```python
from build123d import *

# Parameters (mm, degrees)
SKETCH1_R           = 1.4
BOSS_EXTRUDE1_DEPTH = 0.8


with BuildPart() as part:
    # Sketch1 → Boss-Extrude1 (new, symmetric)
    with BuildSketch(Plane(origin=(0, 0, 0), x_dir=(0, 0, -1), z_dir=(1, 0, 0))):
        with BuildLine():
            Line((-35.297434934, -41.688153), (-20.809434934, -41.688153))
            Line((-20.809434934, -41.688153), (-20.809434934, -39.097053))
            Line((-20.809434934, -39.097053), (14.496565066, -39.097053))
            Line((14.496565066, -39.097053), (14.496565066, -41.688153))
            Line((14.496565066, -41.688153), (34.592039339, -41.688153))
            ThreePointArc((34.592039339, -41.688153), (38.127573245, -40.223686906), (39.592039339, -36.688153))
            Line((39.592039339, -36.688153), (39.592039339, 35.784769822))
            ThreePointArc((39.592039339, 35.784769822), (38.127573245, 39.320303728), (34.592039339, 40.784769822))
            Line((34.592039339, 40.784769822), (-29.297434934, 40.784769822))
            Line((-29.297434934, 40.784769822), (-29.297434934, 33.728413265))
            ThreePointArc((-29.297434934, 33.728413265), (-30.029667981, 31.960646312), (-31.797434934, 31.228413265))
            Line((-31.797434934, 31.228413265), (-40.297434934, 31.228413265))
            Line((-40.297434934, 31.228413265), (-40.297434934, -36.688153))
            ThreePointArc((-40.297434934, -36.688153), (-38.83296884, -40.223686906), (-35.297434934, -41.688153))
        make_face()
        with Locations((-36.797434934, 27.284769822)):
            Circle(SKETCH1_R, mode=Mode.SUBTRACT)
        with Locations((21.202565066, 26.984769822)):
            Circle(SKETCH1_R, mode=Mode.SUBTRACT)
        with Locations((-35.297434934, -34.715230178)):
            Circle(SKETCH1_R, mode=Mode.SUBTRACT)
        with Locations((35.202565066, -34.715230178)):
            Circle(SKETCH1_R, mode=Mode.SUBTRACT)
    extrude(amount=BOSS_EXTRUDE1_DEPTH, both=True)


solid = part.part
```
The model under review builds one solid part; all positions refer to its coordinate system, in mm. Round coordinates to 2 decimals unless told otherwise and drop trailing zeros. Write each loop counter-clockwise with the first axis right and the second up, starting at its lowest first coordinate (ties: lowest second). Pieces come first, ordered by that corner, then holes. Notation, with made-up numbers: (7.5, -8) - (54.5, -8) arc R6 cw to (54.5, 0) - close; hole circle Ø1 at (26, 7.5). An arc over 180 degrees is marked (long way). Answer as CSV lines item,"result". Start each with the question number.
(1) For pin 1 Ø6 at (y, z) = (27, -21.5) entering from +X; pin 2 Ø0.5 at (x, z) = (0, -2.5) entering from -Y; pin 3 Ø1.7 at (y, z) = (26.98, -21.2) entering from -X, all flat-tipped, find the tip position at first contact; note any pin that passes through.
(2) To check wall thickness, follow line 1 (Y direction, x = -0.4, z = -35); line 2 (Y direction, x = 0, z = -13); line 3 (Y direction, x = 0.25, z = 34.5). State the ranges of each line that lie inside material, in increasing order.
(3) We need section B-B on x = 0.4. State the section outline as (y, z) points, plus the area to 3 significant figures.
(4) We need section A-A on z = 1.5. State the section outline as (x, y) points.
(5) Draft analysis for pull direction Z (two halves, no side actions). For faces 1 (the cylindrical face through (-0.011, -34.654, 36.696)), 2 (the flat face through (-0.8, 0, 1)), 3 (the cylindrical face through (0.01, -40.26, -38.09)), 4 (the cylindrical face through (-0.011, 25.743, -21.849)), state which applies: pulls with the +Z half, pulls with the -Z half, needs draft (parallel to the pull), parting line crosses it, or undercut.
Worked answers:
1,pin 1,"x = 0.8"
1,pin 2,"y = -39.1"
1,pin 3,"through"
2,line 1,"-41.67 to -36.1, -33.33 to 40.77"
2,line 2,"-39.1 to 40.78"
2,line 3,"-41.69 to -35.87, -33.56 to 31.23"
3,outline,"(-41.69, -34.59) arc R5 ccw to (-36.69, -39.59) - (35.78, -39.59) arc R5 ccw to (40.78, -34.59) - (40.78, 29.3) - (33.73, 29.3) arc R2.5 cw to (31.23, 31.8) - (31.23, 40.3) - (-36.69, 40.3) arc R5 ccw to (-41.69, 35.3) - (-41.69, 20.81) - (-39.1, 20.81) - (-39.1, -14.5) - (-41.69, -14.5) - close; hole circle Ø2.8 at (-34.72, -35.2); hole circle Ø2.8 at (-34.72, 35.3); hole circle Ø2.8 at (26.98, -21.2); hole circle Ø2.8 at (27.28, 36.8)"
3,area,"6,350 mm²"
4,outline,"(-0.8, -39.1) - (0.8, -39.1) - (0.8, 40.78) - (-0.8, 40.78) - close"
5,face 1,"undercut"
5,face 2,"needs draft"
5,face 3,"pulls with the -Z half"
5,face 4,"undercut"
